Build history of the part. All positions in model axes, mm. Round coordinates to 2 decimals unless told otherwise and drop trailing zeros. Loops run counter-clockwise (first coordinate to the right, second up) from the corner with the lowest first, then second, coordinate; pieces in that order, holes last. Notation, with made-up numbers: M 25.25,34 L 57.25,34 A21 ccw 57.25,44 Z; hole C 10,48.25 d4. An arc over 180 degrees is marked long. One line per item, written item: value.
```python
from build123d import *

# Parameters (mm, degrees)
BOSS_EXTRU_1_DEPTH                = 5
DIAM_TRE_DU_PER_AGE_5_0_5_1_D     = 5
DIAM_TRE_DU_PER_AGE_5_0_5_1_DEPTH = 5


with BuildPart() as part:
    # Esquisse1 → Boss.-Extru.1 (new body)
    with BuildSketch(Plane.XY):
        Polygon((0, 66), (5, 66), (5, 0), (245, 0), (245, 66), (250, 66), (250, 132), (245, 132), (245, 198), (250, 198), (250, 264), (245, 264), (245, 330), (197, 330), (197, 325), (149, 325), (149, 330), (101, 330), (101, 325), (53, 325), (53, 330), (5, 330), (5, 264), (0, 264), (0, 198), (5, 198), (5, 132), (0, 132), align=None)
    extrude(amount=BOSS_EXTRU_1_DEPTH)

    # Diamètre du perçage Ø5.0 (5)1
    with Locations(Plane.XY.offset(5)):
        with Locations((35, 295), (215, 295), (215, 100), (35, 100)):
            Hole(DIAM_TRE_DU_PER_AGE_5_0_5_1_D / 2, depth=DIAM_TRE_DU_PER_AGE_5_0_5_1_DEPTH)


solid = part.part
```
Item 1: Slice it at B-B, the plane x = 68.5. Give the cut face in (y, z).
Check values:
outline: M 0,0 L 325,0 L 325,5 L 0,5 Z
Item 2: Drop flat-ended pins along their axis: P1, Ø1.5, axis at y = 22, z = 3.5, coming from the -X side; P2, Ø4, axis at x = 215, y = 295, coming from the -Z side; P3, Ø2, axis at x = 170.5, z = 3.5, coming from the -Y side; P4, Ø2.5, axis at x = 2, z = 2, coming from the +Y side. Give the stop position or say it passes through.
Check values:
P1: stops at x = 5
P2: passes through
P3: stops at y = 0
P4: stops at y = 264
Item 3: Wall check: line 1 along Y through (x, z) = (35, 3.05); line 2 along X through (y, z) = (295, 1.9); line 3 along Y through (x, z) = (80, 0.6). Give the ranges that are in metal, low to high.
Check values:
line 1: y = 0 to 97.5, 102.5 to 292.5, 297.5 to 330
line 2: x = 5 to 32.5, 37.5 to 212.5, 217.5 to 245
line 3: y = 0 to 325
Item 4: Slice it at C-C, the plane y = 279. Give the cut face in (x, z).
Check values:
outline: M 5,0 L 245,0 L 245,5 L 5,5 Z
Item 5: Slice it at A-A, the plane z = 2.7. Give the number of separate pieces and of enclosed holes in the cut face, and give its area (3 significant figures).
Check values:
separate pieces: 1
enclosed holes: 4
area: 80,000 mm2
